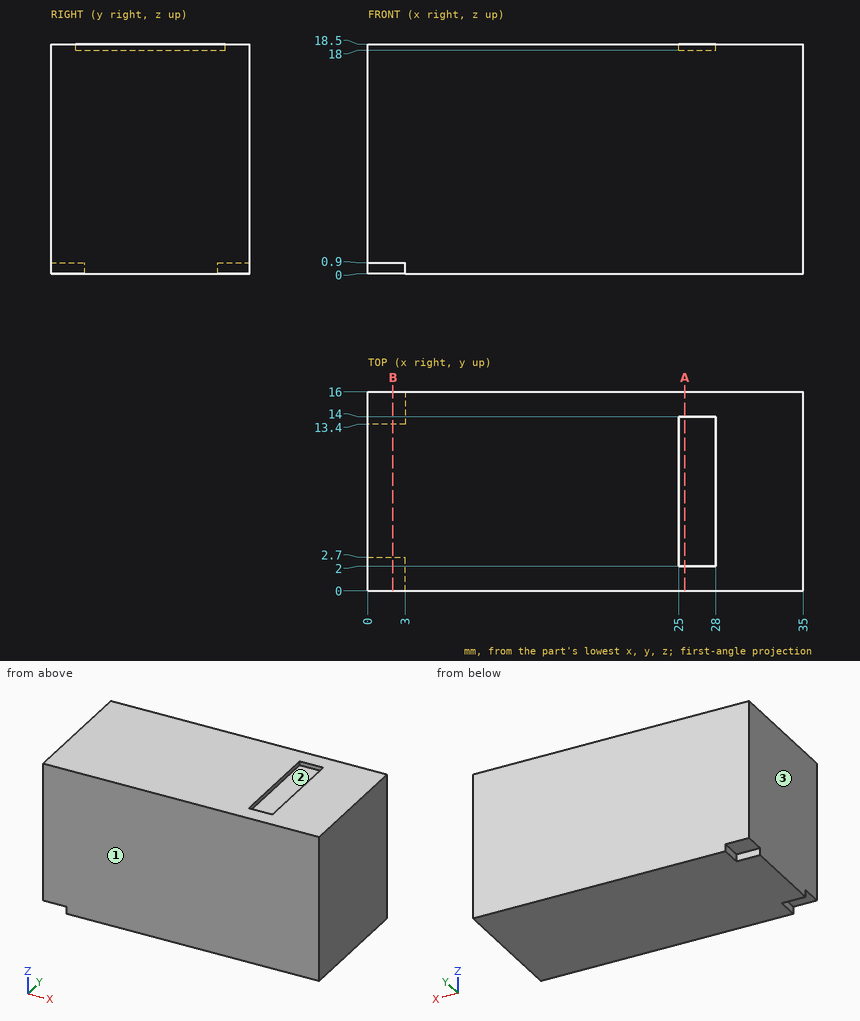
Geometry check sheet. Reference: drawing and pictorial views, mm from the part's lowest x, y, z. Round coordinates to 2 decimals unless told otherwise and drop trailing zeros. Order: outer loops, then holes, each group sorted by start corner. A loop starts at its lowest first (then second) coordinate and runs counter-clockwise, first axis right, second up. Notation, with made-up numbers: (37.5, -17.75) - (85.5, -17.75) arc R32 cw to (85.5, 11.25) - close; hole circle Ø9 at (49, 7.5). An arc over 180 degrees is marked (long way). One line per question, with ' | ' between items. Start each with the question number.
(1) Sectioned sample at A-A on x = 25.5. Record the cut outline in (y, z).
(2) Release check for a two-part mould opening along Y. For the marked faces 1, 2 and 3 record: released by +Y, released by -Y, zero draft, split by the parting line, or undercut.
(3) Depth check by flat-ended pin: pin 1 Ø0.5 at (y, z) = (2, 0.5) entering from -X; pin 2 Ø0.8 at (x, y) = (1.5, 14.5) entering from -Z. Enter the tip coordinate at first touch or a pass-through.
(4) Sectioned sample at B-B on x = 2. Record the cut outline in (y, z).
Conclusion:
1) outline: (0, 0) - (16, 0) - (16, 18.5) - (14, 18.5) - (14, 18) - (2, 18) - (2, 18.5) - (0, 18.5) - close
2) face 1: released by -Y | face 2: undercut | face 3: zero draft
3) pin 1: stops at x = 3 | pin 2: stops at z = 0.9
4) outline: (0, 0.9) - (2.7, 0.9) - (2.7, 0) - (13.4, 0) - (13.4, 0.9) - (16, 0.9) - (16, 18.5) - (0, 18.5) - close
